```python
from build123d import *

# Parameters (mm, degrees)
SKETCH1_W           = 104
SKETCH1_H           = 104
BOSS_EXTRUDE1_DEPTH = 57.5
CUT_EXTRUDE1_DEPTH  = 104
CUT_EXTRUDE2_DEPTH  = 104
SKETCH4_R           = 25
CUT_EXTRUDE3_DEPTH  = 115
SKETCH5_R           = 35
SKETCH5_R_2         = 25
CUT_EXTRUDE4_DEPTH  = 10
CUT_EXTRUDE5_START  = -10
SKETCH6_R           = 35
CUT_EXTRUDE5_DEPTH  = 10
SKETCH7_W           = 52
SKETCH7_H           = 52
CUT_EXTRUDE6_DEPTH  = 115
FILLET1_R           = 15
BOSS_EXTRUDE2_DEPTH = 10
CUT_EXTRUDE7_DEPTH  = 10
FILLET2_R           = 5


with BuildPart() as part:
    # Sketch1 → Boss-Extrude1 (new, symmetric)
    with BuildSketch(Plane(origin=(0, 0, 0), x_dir=(1, 0, 0), z_dir=(0, 1, 0))):
        with Locations((52, 52)):
            Rectangle(SKETCH1_W, SKETCH1_H)
    extrude(amount=BOSS_EXTRUDE1_DEPTH, both=True)

    # Sketch2 → Cut-Extrude1 (cut)
    with BuildSketch(Plane.XY):
        Polygon((0, -57.5), (24.407301932, 0), (0, 57.5), align=None)
        Polygon((104, 57.5), (79.592698068, 0), (104, -57.5), align=None)
    extrude(amount=-CUT_EXTRUDE1_DEPTH, mode=Mode.SUBTRACT)

    # Sketch3 → Cut-Extrude2 (cut)
    with BuildSketch(Plane.ZY.offset(-104)):
        Polygon((-104, 57.5), (-79.592698068, 0), (-104, -57.5), align=None)
        Polygon((0, 57.5), (-24.407301932, 0), (0, -57.5), align=None)
    extrude(amount=CUT_EXTRUDE2_DEPTH, mode=Mode.SUBTRACT)

    # Sketch4 → Cut-Extrude3 (cut)
    with BuildSketch(Plane(origin=(0, 57.5, 0), x_dir=(1, 0, 0), z_dir=(0, 1, 0))):
        with Locations(Location((52, 52, 0), (0, 0, 270))):
            Circle(SKETCH4_R)
    extrude(amount=-CUT_EXTRUDE3_DEPTH, mode=Mode.SUBTRACT)

    # Sketch5 → Cut-Extrude4 (cut)
    with BuildSketch(Plane(origin=(0, 57.5, 0), x_dir=(1, 0, 0), z_dir=(0, 1, 0))):
        with Locations(Location((52, 52, 0), (0, 0, 270))):
            Circle(SKETCH5_R)
        with Locations(Location((52, 52, 0), (0, 0, 270))):
            Circle(SKETCH5_R_2, mode=Mode.SUBTRACT)
    extrude(amount=-CUT_EXTRUDE4_DEPTH, mode=Mode.SUBTRACT)

    # Sketch6 → Cut-Extrude5 (cut)
    with BuildSketch(Plane.XZ.offset(57.5).offset(CUT_EXTRUDE5_START)):
        with Locations(Location((52, -52, 0), (0, 0, 90))):
            Circle(SKETCH6_R)
    extrude(amount=CUT_EXTRUDE5_DEPTH, mode=Mode.SUBTRACT)

    # Sketch7 → Cut-Extrude6 (cut)
    with BuildSketch(Plane(origin=(0, 57.5, 0), x_dir=(1, 0, 0), z_dir=(0, 1, 0))):
        with Locations((78, 26)):
            Rectangle(SKETCH7_W, SKETCH7_H)
    extrude(amount=-CUT_EXTRUDE6_DEPTH, mode=Mode.SUBTRACT)

    # Fillet1
    fillet1_edges = [part.edges().sort_by_distance(p)[0] for p in [
        (24.407301932, 0, -52),
        (79.592698068, 0, -65.796349034),
        (52, 0, -79.592698068),
        (38.203650966, 0, -24.407301932),
    ]]
    fillet(fillet1_edges, radius=FILLET1_R)

    # Sketch8 → Boss-Extrude2 (add)
    with BuildSketch(Plane(origin=(0, 57.5, 0), x_dir=(1, 0, 0), z_dir=(0, 1, 0))):
        Polygon((101, 101), (101, 52), (104, 52), (104, 104), (0, 104), (0, 0), (52, 0), (52, 3), (3, 3), (3, 101), align=None)
    extrude(amount=BOSS_EXTRUDE2_DEPTH)

    # Sketch9 → Cut-Extrude7 (cut)
    with BuildSketch(Plane(origin=(0, 57.5, 0), x_dir=(1, 0, 0), z_dir=(0, 1, 0))):
        with BuildLine():
            Line((13.462680425, 94.779960262), (24.069282143, 84.173358544))
            ThreePointArc((24.069282143, 84.173358544), (24.069282143, 79.930717857), (19.826641456, 79.930717857))
            Line((19.826641456, 79.930717857), (9.220039738, 90.537319575))
            ThreePointArc((9.220039738, 90.537319575), (9.220039738, 94.779960262), (13.462680425, 94.779960262))
        make_face()
        with BuildLine():
            Line((94.779960262, 90.537319575), (84.173358544, 79.930717857))
            ThreePointArc((84.173358544, 79.930717857), (79.930717857, 79.930717857), (79.930717857, 84.173358544))
            Line((79.930717857, 84.173358544), (90.537319575, 94.779960262))
            ThreePointArc((90.537319575, 94.779960262), (94.779960262, 94.779960262), (94.779960262, 90.537319575))
        make_face()
        with BuildLine():
            Line((24.069282143, 19.826641456), (13.462680425, 9.220039738))
            ThreePointArc((13.462680425, 9.220039738), (9.220039738, 9.220039738), (9.220039738, 13.462680425))
            Line((9.220039738, 13.462680425), (19.826641456, 24.069282143))
            ThreePointArc((19.826641456, 24.069282143), (24.069282143, 24.069282143), (24.069282143, 19.826641456))
        make_face()
    extrude(amount=-CUT_EXTRUDE7_DEPTH, mode=Mode.SUBTRACT)

    # Fillet2
    fillet2_edges = [part.edges().sort_by_distance(p)[0] for p in [
        (104, 57.5, -78),
        (3, 57.5, -52),
        (52, 57.5, -104),
        (26, 57.5, 0),
    ]]
    fillet(fillet2_edges, radius=FILLET2_R)


solid = part.part
```
Input: part model. Units: mm. Frame: model coordinates. A direction names the side the tool comes from. Give positions to 0.01 mm unless a question says otherwise; leave off trailing zeros. Order: outer loops, then holes, each group sorted by start corner. A loop starts at its lowest first (then second) coordinate and runs counter-clockwise, first axis right, second up. Notation, with made-up numbers: (-3.5, 27) - (47.5, 27) arc R15 cw to (47.5, 36) - close; hole circle Ø6 at (82.25, 36.5). An arc over 180 degrees is marked (long way). Use a Markdown table: item, result.
(1) Section query B-B (x = 64). Output: boundary loops of the cut face in (y, z).
Computed values:
| item | result |
|---|---|
| outline | (-57.5, -104) - (-5.86, -82.08) arc R15 cw to (5.86, -82.08) - (56.56, -103.6) arc R5 ccw to (58.52, -104) - (67.5, -104) - (67.5, -101) - (57.5, -101) - (57.5, -84.88) - (47.5, -84.88) - (47.5, -73.93) - (-47.5, -73.93) - (-47.5, -84.88) - (-57.5, -84.88) - close |
(2) Line query: line 1 (Y direction, x = 80, z = -74); line 2 (Y direction, x = 96.5, z = -74.5); line 3 (Y direction, x = 90, z = -87). Output: solid intervals per line, ascending. Write a range as from..to.
Computed values:
| item | result |
|---|---|
| line 1 | y = -57.5..57.5 |
| line 2 | y = -57.5..-39.83, 39.83..57.5 |
| line 3 | y = -57.5..-24.52, 24.52..47.5 |
(3) Access query for faces 4 (the flat face through (34, -47.5, -70)), 5 (the flat face through (104, 63, -78)), 6 (the flat face through (51, 62, -101)), 7 (the flat face through (52.722, 31.567, -92.992)), 8 (the flat face through (92.992, 31.567, -71.706)). Directions: +Z, -Z, +X, -X, +Y, -Y. A direction counts if a zero-diameter tool reaches every point of the face in a straight line with its end or side. Return the directions, or none.
Computed values:
| item | result |
|---|---|
| face 4 | -Y |
| face 5 | +Z, -Z, +X, +Y, -Y |
| face 6 | +Y |
| face 7 | -Z, +X, -X |
| face 8 | +Z, -Z, +X |
(4) Section query C-C (y = 32.5). Output: boundary loops of the cut face in (x, z), then the cut area to 3 significant figures.
Computed values:
| item | result |
|---|---|
| outline | (10.61, -93.39) - (93.39, -93.39) - (93.39, -52) - (77, -52) arc R25 cw (long way) to (52, -27) - (52, -10.61) - (10.61, -10.61) - close |
| area | 3,670 mm2 |
(5) Section query D-D (y = -2). Output: boundary loops of the cut face in (x, z), then the cut area to 3 significant figures.
Computed values:
| item | result |
|---|---|
| outline | (22.98, -81.02) - (81.02, -81.02) - (81.02, -52) - (77, -52) arc R25 cw (long way) to (52, -27) - (52, -22.98) - (22.98, -22.98) - close |
| area | 1,050 mm2 |
(6) Draft query along Y for faces 1 (the flat face through (52, 5.9, -22.3)), 2 (the flat face through (17, 47.5, -17)), 3 (the flat face through (52.728, -31.319, -92.887)). Return one class per face: released by +Y, released by -Y, zero draft, split by the parting line, or undercut.
Computed values:
| item | result |
|---|---|
| face 1 | zero draft |
| face 2 | released by +Y |
| face 3 | undercut |
(7) Section query A-A (z = -43.5). Output: boundary loops of the cut face in (x, y), then the cut area to 3 significant figures.
Computed values:
| item | result |
|---|---|
| outline | (0, -57.5) - (18.05, -57.5) - (18.05, -47.5) - (28.49, -47.5) - (28.49, 47.5) - (18.05, 47.5) - (18.05, 57.5) - (8, 57.5) arc R5 cw to (3, 62.5) - (3, 67.5) - (0, 67.5) - (0, 57.5) - (21.92, 5.86) arc R15 cw to (21.92, -5.86) - close |
| area | 1,700 mm2 |
(8) Pin query (flat end, axial travel): pin 1 (3 mm diameter, centred on y = -40, z = -92.5, fed in from -X); pin 2 (12 mm diameter, centred on x = 42, y = 50, fed in from +Z); pin 3 (1 mm diameter, centred on y = -17.5, z = -59, fed in from +X). Return the tip coordinate at first contact, or that it passes through.
Computed values:
| item | result |
|---|---|
| pin 1 | stops at x = 6.79 |
| pin 2 | stops at z = -0.64 |
| pin 3 | stops at x = 87.23 |
